from build123d import *

# Parameters (mm, degrees)
F0_W     = 21
F0_H     = 15
F0_W_2   = 19.5
F0_H_2   = 12.75
F1_DEPTH = 22
F0_R     = 1.7
F2_DEPTH = 2
F3_R     = 3.4
F5_DEPTH = 18


with BuildPart() as f1:
    # F0 (on Top) → F1 (new body)
    with BuildSketch(Plane.XY):
        Rectangle(F0_W, F0_H)
        Rectangle(F0_W_2, F0_H_2, mode=Mode.SUBTRACT)
        Rectangle(F0_W_2, F0_H_2)
    extrude(amount=F1_DEPTH)

    # F0 (on Top) → F2 (join)
    with BuildSketch(Plane.XY):
        Polygon((10.5, -7.5), (-10.5, -7.5), (0, -17.5), align=None)
        with Locations((0, -12.5)):
            Circle(F0_R, mode=Mode.SUBTRACT)
        Polygon((0, 17.5), (-10.5, 7.5), (10.5, 7.5), align=None)
        with Locations((0, 12.5)):
            Circle(F0_R, mode=Mode.SUBTRACT)
    extrude(amount=F2_DEPTH)

    # F3
    f3_edges = [f1.edges().sort_by_distance(p)[0] for p in [
        (0, -17.5, 1),
        (0, 17.5, 1),
    ]]
    fillet(f3_edges, radius=F3_R)

    # F4 (on face) → F5 (cut)
    with BuildSketch(Plane.XY.offset(22)):
        Polygon((-4, -7.5), (0, -7.5), (4, -7.5), (4, 7.5), (-4, 7.5), align=None)
    extrude(amount=-F5_DEPTH, mode=Mode.SUBTRACT)


solid = f1.part
Can you work these out from the model? Positions are in its coordinate system, mm. A direction names the side the tool comes from. Round coordinates to 2 decimals unless told otherwise and drop trailing zeros. Write each loop counter-clockwise with the first axis right and the second up, starting at its lowest first coordinate (ties: lowest second). Pieces come first, ordered by that corner, then holes. Notation, with made-up numbers: M 20,80.25 L 79,80.25 A17 cw 79,113.25 Z; hole C -25,6.5 d6. An arc over 180 degrees is marked long. Use CSV: the item, a comma, the result in double quotes.
(1) Imagine slicing it at D-D (y = -4). Write out the boundary of the cut face in (x, z).
Check values:
outline,"M -10.5,0 L 10.5,0 L 10.5,22 L 4,22 L 4,4 L -4,4 L -4,22 L -10.5,22 Z"
(2) On a 3-axis mill with a long thin cutter (end or side, diameter ignored), from which of +Z, -Z, +X, -X, +Y, -Y can I reach the whole of each face in a straight line? I mean faces 1 (the flat face through (4, 0, 13)), 2 (the flat face through (6.48, 11.33, 0.99)), 3 (the flat face through (10.5, 0, 11)), 4 (the flat face through (-5, -7.5, 12)), 5 (the flat face through (-5, 7.5, 12)). Say none if no direction works.
Check values:
face 1,"+Z, +Y, -Y"
face 2,"+Z, -Z, +X, +Y"
face 3,"+Z, -Z, +X, +Y, -Y"
face 4,"+Z, +X, -X, -Y"
face 5,"+Z, +X, -X, +Y"
(3) Imagine slicing it at A-A (z = 17). Write out the boundary of the cut face in (x, y).
Check values:
outline,"M -10.5,-7.5 L -4,-7.5 L -4,7.5 L -10.5,7.5 Z; M 4,-7.5 L 10.5,-7.5 L 10.5,7.5 L 4,7.5 Z"
(4) Imagine slicing it at C-C (y = -12.5). Write out the boundary of the cut face in (x, z).
Check values:
outline,"M -5.25,0 L -1.7,0 L -1.7,2 L -5.25,2 Z; M 1.7,0 L 5.25,0 L 5.25,2 L 1.7,2 Z"
(5) We'd pull the mould along X, two halves only. Please class faces 6 (the cylindrical face through (-0.221, -10.814, 0.986)), 7 (the flat face through (-7, 0, 22)), 8 (the flat face through (-4, 0, 13)), 9 (the flat face through (-6.48, -11.33, 0.99)): +X half, -X half, draft (parallel to the pull), parting line (faces both ways), or undercut.
Check values:
face 6,"undercut"
face 7,"draft"
face 8,"undercut"
face 9,"-X half"
(6) I need wall thicknesses on line 1 along Y through (x, z) = (0, 1.55); line 2 along X through (y, z) = (-2, 16.75); line 3 along Z through (x, y) = (-5, -9.5). Which ranges of each line are inside material? Lowest first, please.
Check values:
line 1,"-16.2 to -14.2, -10.8 to 10.8, 14.2 to 16.2"
line 2,"-10.5 to -4, 4 to 10.5"
line 3,"0 to 2"
(7) I'm going to push flat-ended pins straight in: pin 1 (9.5 mm diameter, centred on x = 2, y = 12, fed in from +Z); pin 2 (2.5 mm diameter, centred on x = 0, y = -12.5, fed in from -Z); pin 3 (1.5 mm diameter, centred on x = -0.5, y = 10, fed in from +Z). Where does each tip first touch, or does it pass through?
Check values:
pin 1,"z = 4"
pin 2,"through"
pin 3,"z = 2"
(8) Imagine slicing it at B-B (x = 0). Write out the boundary of the cut face in (y, z), plus the area to 3 significant figures.
Check values:
outline,"M -16.2,0 L -14.2,0 L -14.2,2 L -16.2,2 Z; M -10.8,0 L 10.8,0 L 10.8,2 L 7.5,2 L 7.5,4 L -7.5,4 L -7.5,2 L -10.8,2 Z; M 14.2,0 L 16.2,0 L 16.2,2 L 14.2,2 Z"
area,"81.2 mm^2"
